from build123d import *

# Parameters (mm, degrees)
F1_DEPTH  = 2.25
F2_DEPTH  = 1.1
F3_SIZE   = 0.9
F5_DEPTH  = 12
F6_R      = 1.75
F6_R_2    = 1.25
F7_DEPTH  = 1.7
F8_DEPTH  = 12.001
F9_R      = 0.9
F10_DEPTH = 8.2


with BuildPart() as f1:
    # F0 (on Top) → F1 (new body, symmetric)
    with BuildSketch(Plane.XY):
        Polygon((0, 0), (0, 5), (-12, 5), (-12, 0), (-11.9, 0), (-6.1, 0), align=None)
    extrude(amount=F1_DEPTH, both=True)

    # F0 (on Top) → F2 (join, symmetric)
    with BuildSketch(Plane.XY):
        Polygon((-6.1, -3.996311), (-6.1, 0), (-11.9, 0), (-11.9, -3.996311), (-11.5187, -4.377611), (-11.104953, -3.963864), (-10.478758, -4.590059), (-10.032431, -4.143733), (-9.488082, -4.688082), (-9, -4.2), (-8.511918, -4.688082), (-7.967569, -4.143733), (-7.521242, -4.590059), (-6.895047, -3.963864), (-6.4813, -4.377611), align=None)
    extrude(amount=F2_DEPTH, both=True)

    # F3
    f3_edges = [f1.edges().sort_by_distance(p)[0] for p in [
        (-6, 0, 2.25),
        (-6, 0, -2.25),
    ]]
    chamfer(f3_edges, length=F3_SIZE)

    # F4 (on Right) → F5 (cut)
    with BuildSketch(Plane.YZ):
        Polygon((-4.9, 0.52265), (-3.9, 1.1), (-4.9, 1.1), align=None)
        Polygon((-4.9, -1.1), (-3.9, -1.1), (-4.9, -0.52265), align=None)
    extrude(amount=-F5_DEPTH, mode=Mode.SUBTRACT)

    # F6 (on face) → F7 (join)
    with BuildSketch(Plane(origin=(-12, 0, 0), x_dir=(0, -1, 0), z_dir=(-1, 0, 0))):
        with Locations((-2.3, 0)):
            Circle(F6_R)
        with Locations((-2.3, 0)):
            Circle(F6_R_2, mode=Mode.SUBTRACT)
    extrude(amount=F7_DEPTH)

    # F6 (on face) → F8 (cut, through all)
    with BuildSketch(Plane(origin=(-12, 0, 0), x_dir=(0, -1, 0), z_dir=(-1, 0, 0))):
        with Locations((-2.3, 0)):
            Circle(F6_R_2)
    extrude(amount=-F8_DEPTH, mode=Mode.SUBTRACT)

    # F9 (on face) → F10 (cut)
    with BuildSketch(Plane(origin=(0, 5, 0), x_dir=(-1, 0, 0), z_dir=(0, 1, 0))):
        with Locations((9.5, 0)):
            Circle(F9_R)
    extrude(amount=-F10_DEPTH, mode=Mode.SUBTRACT)


solid = f1.part
Verification items for the finished model (mm, model axes). A direction names the side the tool comes from. Coordinates: 2 decimals unless noted, no trailing zeros. Order: outer loops, then holes, each group sorted by start corner. A loop starts at its lowest first (then second) coordinate and runs counter-clockwise, first axis right, second up. Notation, with made-up numbers: (14.5, -39.5) -> (30.5, -39.5) arc R28 ccw to (30.5, -1.5) -> close; hole circle Ø4 at (21.5, 42.5). An arc over 180 degrees is marked (long way). Put each result on its own line as item: value. Start each with the question number.
1. Cross-section at B-B, the plane x = -2. Record the boundary of the cut face in (y, z), then the cut area to 3 significant figures.
2. Mould release check, pull along X, two halves, no side actions. Record for faces 4 (the flat face through (-9, -3.2, 0)), 5 (the flat face through (-12, 4.2, 0)), 6 (the flat face through (-9, -2, -1.1)): released by +X, released by -X, zero draft, split by the parting line, or undercut.
3. Go/stop test with flat-tipped pins: pin 1 Ø2 at (x, y) = (-9.5, -2.5) entering from -Z; pin 2 Ø1.4 at (x, z) = (-9.5, 0) entering from +Y; pin 3 Ø2 at (x, y) = (-8.5, -2) entering from +Z. Record where each tip stops, or that it passes through.
4. Material ranges on L1, parallel to X at y = -2, z = 0; L2, parallel to Y at x = -4, z = -0.1; L3, parallel to Z at x = -13, y = 2.3, recorded low to high. Write a range as [from, to].
5. Cross-section at A-A, the plane y = 2.3. Record the boundary of the cut face in (x, z).
6. Cross-section at D-D, the plane y = -3.75. Record the boundary of the cut face in (x, z).
7. Cross-section at C-C, the plane z = 0. Count the separate pieces of the cut face and the enclosed holes in it, then the cut area to 3 significant figures.
8. Access from +Z, -Z, +X, -X, +Y, -Y to the whole of each face (thin tool, end or side, straight path). Record for faces 1 (the flat face through (-9, -2, 1.1)), 2 (the cylindrical face through (-9.38, -0.85, 0.89)), 3 (the flat face through (-6.1, -2, 0)).
Computed:
1. outline: (0, -1.35) -> (0.9, -2.25) -> (5, -2.25) -> (5, 2.25) -> (0.9, 2.25) -> (0, 1.35) -> close; hole circle Ø2.5 at (2.3, 0)
1. area: 16.8 mm2
2. face 4: undercut
2. face 5: released by -X
2. face 6: zero draft
3. pin 1: z = -1.1
3. pin 2: y = -3.2
3. pin 3: z = 1.1
4. L1: [-11.9, -10.4], [-8.6, -6.1]
4. L2: [0, 1.05], [3.55, 5]
4. L3: [-1.75, -1.25], [1.25, 1.75]
5. outline: (-13.7, -1.75) -> (-12, -1.75) -> (-12, -2.25) -> (0, -2.25) -> (0, -1.25) -> (-13.7, -1.25) -> close; (-13.7, 1.25) -> (0, 1.25) -> (0, 2.25) -> (-12, 2.25) -> (-12, 1.75) -> (-13.7, 1.75) -> close
6. outline: (-11.9, -1.1) -> (-6.1, -1.1) -> (-6.1, 1.1) -> (-11.9, 1.1) -> close
7. separate pieces: 3
7. enclosed holes: 0
7. area: 46.5 mm2
8. face 1: +Z, +X, -X, -Y
8. face 2: +Y
8. face 3: +Z, -Z, +X, -Y
